Can you work these out from the model? Positions are in its coordinate system, mm. Face numbers are marked on the shaded views. A direction names the side the tool comes from. Give positions to 0.01 mm unless a question says otherwise; leave off trailing zeros. Order: outer loops, then holes, each group sorted by start corner. A loop starts at its lowest first (then second) coordinate and runs counter-clockwise, first axis right, second up. Notation, with made-up numbers: (87.5, -2.75) - (133.5, -2.75) arc R20 ccw to (133.5, 16.25) - close; hole circle Ø6 at (62.25, 73). An arc over 180 degrees is marked (long way). Write each question's results on one line, items separated by ' | '. Start each with the question number.
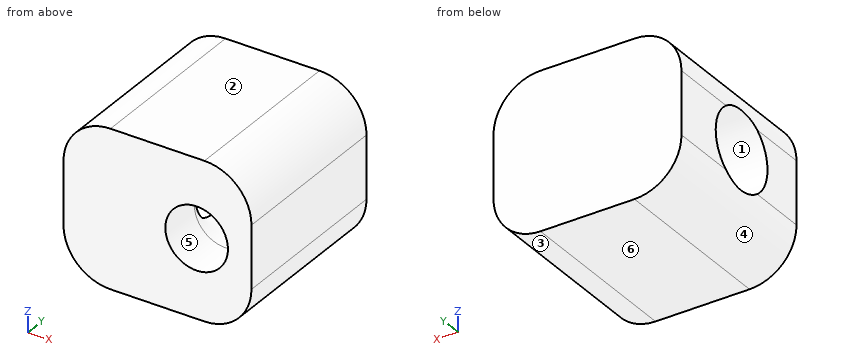
from build123d import *

# Parameters (mm, degrees)
BOSS_EXTRUDE1_DEPTH     = 10
CUT_EXTRUDE2_DEPTH      = 50.456381745
CUT_EXTRUDE2_DEPTH_BACK = 50.456381745
SKETCH3_R               = 2.5
CUT_EXTRUDE3_DEPTH      = 6
SKETCH4_R               = 2
CUT_REVOLVE1_ANGLE      = 90
SKETCH5_R               = 2
CUT_EXTRUDE4_DEPTH      = 2.805452299
FILLET1_R               = 5
SKETCH6_W               = 10
SKETCH6_H               = 29.685485307
CUT_EXTRUDE5_DEPTH      = 33
SKETCH7_W               = 19.76767366
SKETCH7_H               = 10
CUT_EXTRUDE6_DEPTH      = 48.418220859
FILLET2_R               = 3


with BuildPart() as part:
    # Sketch1 → Boss-Extrude1 (new body)
    with BuildSketch(Plane.XY):
        with BuildLine():
            Line((0, 0), (45, 0))
            Line((45, 0), (45, 11.1125))
            Line((45, 11.1125), (35, 11.1125))
            add(Edge.make_bspline(
                [(10, 11.1125), (14.576625097, 20.181995974), (30.423374903, 20.181995974), (35, 11.1125)],
                knots=[0, 0, 0, 0, 1, 1, 1, 1], degree=3))
            Line((10, 11.1125), (0, 11.1125))
            Line((0, 11.1125), (0, 0))
        make_face()
    extrude(amount=-BOSS_EXTRUDE1_DEPTH)

    # Sketch2 → Cut-Extrude2 (cut, two sides: drawn at the far end of the back side and taken through both)
    with BuildSketch(Plane.XY.offset(-CUT_EXTRUDE2_DEPTH_BACK)):
        with BuildLine():
            Line((33, 0), (33, 10.610904597))
            add(Edge.make_bspline(
                [(33, 10.610904597), (32.518518069, 11.455367364), (31.27134268, 12.982349636), (27.931157473, 15.20113612), (22.5, 16.390279221), (17.068842527, 15.20113612), (13.72865732, 12.982349636), (12.481481931, 11.455367364), (12, 10.610904597)],
                knots=[0.018308459, 0.018308459, 0.018308459, 0.018308459, 0.138731344, 0.25915423, 0.5, 0.74084577, 0.861268656, 0.981691541, 0.981691541, 0.981691541, 0.981691541], degree=3))
            Line((12, 10.610904597), (12, 0))
            Line((12, 0), (33, 0))
        make_face()
    extrude(amount=CUT_EXTRUDE2_DEPTH + CUT_EXTRUDE2_DEPTH_BACK, mode=Mode.SUBTRACT)

    # Sketch3 → Cut-Extrude3 (cut)
    with BuildSketch(Plane(origin=(12, 0, 0), x_dir=(0, 0, -1), z_dir=(1, 0, 0))):
        with Locations(Location((5, 5.305452299, 0), (0, 0, 90))):
            Circle(SKETCH3_R)
    cut_extrude3 = extrude(amount=-CUT_EXTRUDE3_DEPTH, mode=Mode.SUBTRACT)

    # Sketch4 → Cut-Revolve1 (revolve, cut)
    with BuildSketch(Plane(origin=(6, 0, 0), x_dir=(0, 0, -1), z_dir=(1, 0, 0))):
        with Locations((5, 5.305452299)):
            Circle(SKETCH4_R)
    cut_revolve1 = revolve(axis=Axis((6, 2.805452299, -5), (0, 0, 1)), revolution_arc=CUT_REVOLVE1_ANGLE, mode=Mode.SUBTRACT)

    # Sketch5 → Cut-Extrude4 (cut)
    with BuildSketch(Plane(origin=(0, 2.805452299, 0), x_dir=(1, 0, 0), z_dir=(0, 1, 0))):
        with Locations(Location((3.5, 5, 0), (0, 0, 180))):
            Circle(SKETCH5_R)
    cut_extrude4 = extrude(amount=-CUT_EXTRUDE4_DEPTH, mode=Mode.SUBTRACT)

    # Mirror1: Cut-Extrude3, Cut-Revolve1, Cut-Extrude4 across plane
    add(cut_extrude3.mirror(Plane(origin=(22.5, 0, 0), x_dir=(0, 0, 1), z_dir=(1, 0, 0))), mode=Mode.SUBTRACT)
    add(cut_revolve1.mirror(Plane(origin=(22.5, 0, 0), x_dir=(0, 0, 1), z_dir=(1, 0, 0))), mode=Mode.SUBTRACT)
    add(cut_extrude4.mirror(Plane(origin=(22.5, 0, 0), x_dir=(0, 0, 1), z_dir=(1, 0, 0))), mode=Mode.SUBTRACT)

    # Fillet1
    fillet1_edges = [part.edges().sort_by_distance(p)[0] for p in [
        (10, 11.1125, -5),
        (35, 11.1125, -5),
        (33, 10.610904597, -5),
        (12, 10.610904597, -5),
    ]]
    fillet(fillet1_edges, radius=FILLET1_R)

    # Sketch6 → Cut-Extrude5 (cut)
    with BuildSketch(Plane.ZY):
        with Locations((-5, 14.842742654)):
            Rectangle(SKETCH6_W, SKETCH6_H)
    extrude(amount=-CUT_EXTRUDE5_DEPTH, mode=Mode.SUBTRACT)

    # Sketch7 → Cut-Extrude6 (cut, through all)
    with BuildSketch(Plane(origin=(0, 11.1125, 0), x_dir=(1, 0, 0), z_dir=(0, 1, 0))):
        with Locations((35.11616317, 5)):
            Rectangle(SKETCH7_W, SKETCH7_H)
    extrude(amount=CUT_EXTRUDE6_DEPTH, mode=Mode.SUBTRACT)

    # Fillet2
    # the kernel refuses this fillet: 3 mm, written as the material it takes off along each edge
    with BuildSketch(Plane(origin=(45, -7.5, -10), x_dir=(0, 0, 1), z_dir=(0, 1, 0)), Plane(origin=(33, 18.6125, 0), x_dir=(1, 0, 0), z_dir=(0, -1, 0)), Plane(origin=(45, -7.5, 0), x_dir=(-1, 0, 0), z_dir=(0, 1, 0))) as fillet2_piece_1:
        with BuildLine():
            CenterArc((FILLET2_R, -FILLET2_R), FILLET2_R, 90, 90)
            Line((0, -FILLET2_R), (0, 0))
            Line((0, 0), (FILLET2_R, 0))
        make_face()
    extrude(amount=26.1125, mode=Mode.SUBTRACT)
    with BuildSketch(Plane(origin=(33, 18.6125, -10), x_dir=(1, 0, 0), z_dir=(0, -1, 0))) as fillet2_piece_2:
        with BuildLine():
            CenterArc((FILLET2_R, FILLET2_R), FILLET2_R, 180, 90)
            Line((0, FILLET2_R), (0, 0))
            Line((0, 0), (FILLET2_R, 0))
        make_face()
    extrude(amount=26.1125, mode=Mode.SUBTRACT)


solid = part.part
Q1. Thinking about a two-plate mould opening in X: for the marked faces 3, 4, 5 and 6, which applies, released by +X, released by -X, zero draft, split by the parting line, or undercut?
Q2. Which directions (+Z, -Z, +X, -X, +Y, -Y) give clear straight access to the entire face, cutting with the end or side of a thin tool? Please do the marked faces 1 and 2.
Q3. If we section it at C-C (y = 10): Please give me the cut outline in (x, z).
Q4. If we section it at A-A (z = -5.75): Please give me the cut outline in (x, y).
Q5. If we section it at B-B (y = 1.25): Please give me the cut outline in (x, z).
Q6. Will these pins go through, and if not, where does the flat tip stop? P1, Ø3, axis at x = 39.5, z = -2.5, coming from the -Y side; P2, Ø2, axis at y = 8.5, z = -8.5, coming from the +X side; P3, Ø1.5, axis at y = 5.5, z = -8, coming from the -X side.
Q7. If we section it at D-D (z = -3.5): Please give me the cut outline in (x, y).
Q8. If I drill on probe 1 along Z at (x, y) = (41.5, 1); probe 2 along Z at (x, y) = (37.75, 5); probe 3 along Y at (x, z) = (38, -4.75), over which ranges is the centre line in solid material (lowest first)? Write a range as from..to.
Findings below:
1) face 3: released by +X | face 4: released by -X | face 5: undercut | face 6: zero draft
2) face 1: -X | face 2: +Z, +X, -X, +Y, -Y
3) outline: (33, -7) arc R3 ccw to (36, -10) - (42, -10) arc R3 ccw to (45, -7) - (45, -3) arc R3 ccw to (42, 0) - (36, 0) arc R3 ccw to (33, -3) - close
4) outline: (33, 0) - (39.65, 0) - (39.65, 2.81) arc R0.65 ccw to (39, 3.45) - (39, 2.92) - (33, 2.92) - close; (33, 7.69) - (39, 7.69) - (39, 7.16) arc R4.35 cw to (43.35, 2.81) - (43.35, 0) - (45, 0) - (45, 11.11) - (33, 11.11) - close
5) outline: (33, -7) arc R3 ccw to (36, -10) - (42, -10) arc R3 ccw to (45, -7) - (45, -3) arc R3 ccw to (42, 0) - (36, 0) arc R3 ccw to (33, -3) - close; hole circle Ø4 at (41.5, -5)
6) P1: stops at y = 0 | P2: stops at x = 44.96 | P3: stops at x = 33.03
7) outline: (33, 0) - (40.18, 0) - (40.18, 2.81) arc R1.18 ccw to (39, 3.98) - (39, 3.31) - (33, 3.31) - close; (33, 7.31) - (39, 7.31) - (39, 6.63) arc R3.82 cw to (42.82, 2.81) - (42.82, 0) - (45, 0) - (45, 11.11) - (33, 11.11) - close
8) probe 1: z = -10..-7, -3..0 | probe 2: z = -10..-7.48, -2.52..0 | probe 3: y = 0..2.82, 7.79..11.11
